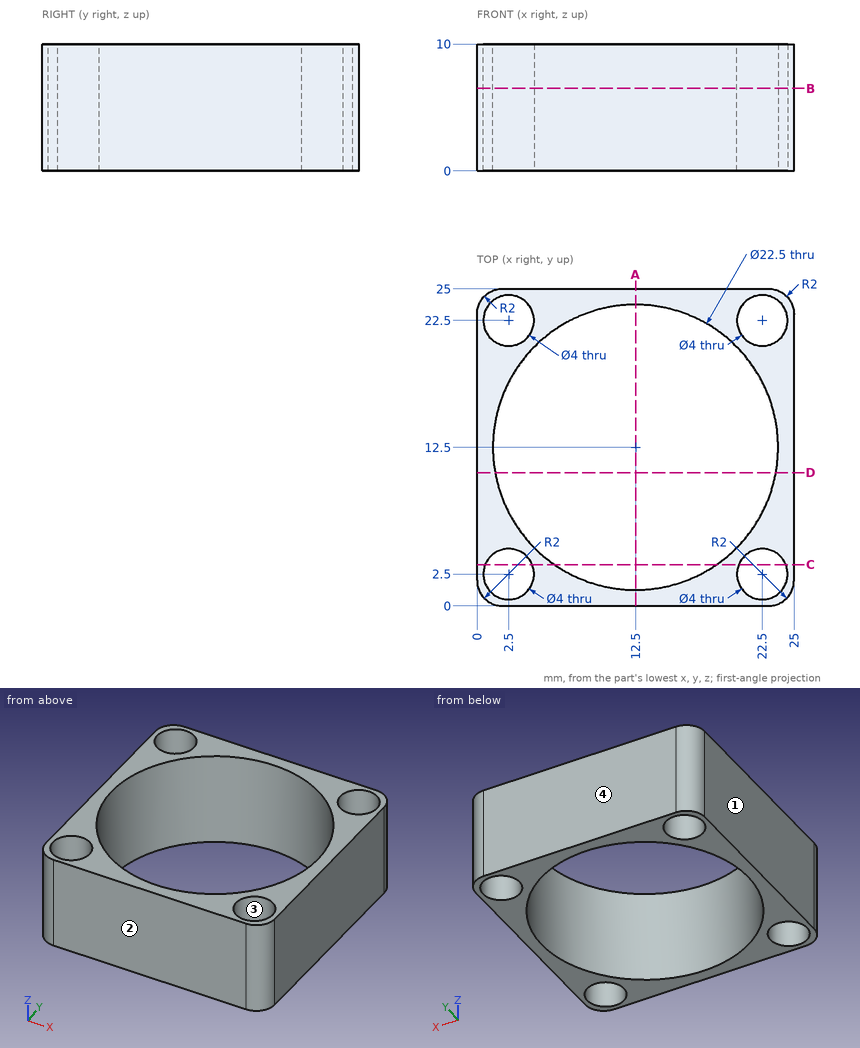
Geometry: see drawing. Coordinates: mm, zero at the bounding-box minimum. Coordinates: 2 decimals unless noted, no trailing zeros. Loops run counter-clockwise (first coordinate to the right, second up) from the corner with the lowest first, then second, coordinate; pieces in that order, holes last. Notation, with made-up numbers: (-33.75, 20) - (-1.75, 20) arc R30 ccw to (-1.75, 51) - close; hole circle Ø7 at (-19, -22). An arc over 180 degrees is marked (long way). Answer as CSV lines item,"result".
1. Section C-C (y = 3.25). Return loops of the section in (x, z).
Established:
outline,"(0, 0) - (0.65, 0) - (0.65, 10) - (0, 10) - close; (4.35, 0) - (6.1, 0) - (6.1, 10) - (4.35, 10) - close; (18.9, 0) - (20.65, 0) - (20.65, 10) - (18.9, 10) - close; (24.35, 0) - (25, 0) - (25, 10) - (24.35, 10) - close"
2. Section B-B (z = 6.5). Return loops of the section in (x, y), then the cut area to 3 significant figures.
Established:
outline,"(0, 2) arc R2 ccw to (2, 0) - (23, 0) arc R2 ccw to (25, 2) - (25, 23) arc R2 ccw to (23, 25) - (2, 25) arc R2 ccw to (0, 23) - close; hole circle Ø4 at (2.5, 2.5); hole circle Ø4 at (2.5, 22.5); hole circle Ø22.5 at (12.5, 12.5); hole circle Ø4 at (22.5, 2.5); hole circle Ø4 at (22.5, 22.5)"
area,"174 mm2"
3. Contact query for a flat-ended pin moving along its axis: pin 1 (1 mm diameter, centred on y = 16, z = 1.5, fed in from -X). Output: stop coordinate, or through.
Established:
pin 1,"stops at x = 0"
4. Section A-A (x = 12.5). Return loops of the section in (y, z), then the cut area to 3 significant figures.
Established:
outline,"(0, 0) - (1.25, 0) - (1.25, 10) - (0, 10) - close; (23.75, 0) - (25, 0) - (25, 10) - (23.75, 10) - close"
area,"25.0 mm2"
5. Ray query, line 1 (Y direction, x = 2.5, z = 4); line 2 (Y direction, x = 21.25, z = 3); line 3 (Y direction, x = 6.5, z = 7.25). Return the intervals inside material, ascending.
Established:
line 1,"y = 0 to 0.5, 4.5 to 7.35, 17.65 to 20.5, 24.5 to 25"
line 2,"y = 0 to 0.94, 4.06 to 5.43, 19.57 to 20.94, 24.06 to 25"
line 3,"y = 0 to 2.98, 22.02 to 25"
6. Mould query, pull axis Y, two halves, no side actions, for the marked faces 1, 2, 3 and 4. Classes: released by +Y, released by -Y, zero draft, split by the parting line, or undercut.
Established:
face 1,"zero draft"
face 2,"released by -Y"
face 3,"undercut"
face 4,"released by +Y"
7. Section D-D (y = 10.5). Return loops of the section in (x, z), then the cut area to 3 significant figures.
Established:
outline,"(0, 0) - (1.43, 0) - (1.43, 10) - (0, 10) - close; (23.57, 0) - (25, 0) - (25, 10) - (23.57, 10) - close"
area,"28.6 mm2"
